The model under review builds one solid part; all positions refer to its coordinate system, in mm. Coordinates: 2 decimals unless noted, no trailing zeros. Write each loop counter-clockwise with the first axis right and the second up, starting at its lowest first coordinate (ties: lowest second). Pieces come first, ordered by that corner, then holes. Notation, with made-up numbers: (41.5, 3) - (89.5, 3) arc R13 cw to (89.5, 17) - close; hole circle Ø3 at (-27, -25). An arc over 180 degrees is marked (long way). Put each result on its own line as item: value.
from build123d import *

# Parameters (mm, degrees)
F0_W      = 48.9472970366
F0_H      = 90.3642401099
F1_DEPTH  = 3.81
F2_R      = 5.08
F3_R      = 1.27
F4_R      = 1.27
F7_W      = 7.0798662491
F7_H      = 0.5429834127
F8_DEPTH  = 0.0254
F10_R     = 2.8950348496
F11_DEPTH = 0.381
F12_R     = 0.254


# Not quite as in the source:
# - the program builds the solid bodies; features that only make, move or delete a surface that nothing else refers to are left out


with BuildPart() as f1:
    # F0 (on Front) → F1 (new body)
    with BuildSketch(Plane.XZ):
        Rectangle(F0_W, F0_H)
    extrude(amount=F1_DEPTH)

    # F2
    f2_edges = [f1.edges().sort_by_distance(p)[0] for p in [
        (-24.473649, -1.905, 45.18212),
        (24.473649, -1.905, 45.18212),
        (24.473649, -1.905, -45.18212),
        (-24.473649, -1.905, -45.18212),
    ]]
    fillet(f2_edges, radius=F2_R)

    # F3
    f3_edges = [f1.edges().sort_by_distance(p)[0] for p in [
        (24.473649, 0, 0),
    ]]
    fillet(f3_edges, radius=F3_R)

    # F4
    f4_edges = [f1.edges().sort_by_distance(p)[0] for p in [
        (0, -3.81, 45.18212),
    ]]
    fillet(f4_edges, radius=F4_R)

    # F7 (on face) → F8 (cut)
    with BuildSketch(Plane.XZ.offset(3.81)):
        with Locations((0, 39.5097658038)):
            Rectangle(F7_W, F7_H)
    extrude(amount=-F8_DEPTH, mode=Mode.SUBTRACT)

    # F10 (on face) → F11 (join)
    with BuildSketch(Plane(origin=(0, 0, 0), x_dir=(-1, 0, 0), z_dir=(0, 1, 0))):
        with Locations((-16.5371242911, 39.8641712964)):
            Circle(F10_R)
    extrude(amount=F11_DEPTH)

    # F12
    f12_edges = [f1.edges().sort_by_distance(p)[0] for p in [
        (19.432159, 0.381, 39.864171),
    ]]
    fillet(f12_edges, radius=F12_R)


solid = f1.part
1. For pin 1 Ø8 at (x, z) = (-9.5, 21) entering from +Y, flat-tipped, find the tip position at first contact; note if it passes through.
Determined:
pin 1: stops at y = 0
2. To check wall thickness, follow probe 1 along Y at (x, z) = (-1, -12); probe 2 along X at (y, z) = (-1.1, -18); probe 3 along Z at (x, y) = (0, -1.2). State the ranges of each line that lie inside material, in increasing order.
Determined:
probe 1: y = -3.81 to 0
probe 2: x = -24.46 to 24.46
probe 3: z = -45.18 to 45.18
3. Consider section A-A on x = -17. State the section outline as (y, z) points.
Determined:
outline: (-3.81, -43.91) arc R1.27 ccw to (-2.54, -45.18) - (-1.27, -45.18) arc R1.27 ccw to (0, -43.91) - (0, 43.91) arc R1.27 ccw to (-1.27, 45.18) - (-2.54, 45.18) arc R1.27 ccw to (-3.81, 43.91) - close
4. Consider section B-B on z = -8.5. State the section outline as (x, y) points, plus the area to 3 significant figures.
Determined:
outline: (-24.47, -2.54) arc R1.27 ccw to (-23.2, -3.81) - (23.2, -3.81) arc R1.27 ccw to (24.47, -2.54) - (24.47, -1.27) arc R1.27 ccw to (23.2, 0) - (-23.2, 0) arc R1.27 ccw to (-24.47, -1.27) - close
area: 185 mm^2
